```python
from build123d import *

# Parameters (mm, degrees)
BOSS_EXTRUDE1_DEPTH = 10
SKETCH2_R           = 10
BOSS_EXTRUDE2_DEPTH = 50
FILLET1_R           = 3
CHAMFER1_SIZE       = 2


with BuildPart() as part:
    # Sketch1 → Boss-Extrude1 (new body)
    with BuildSketch(Plane.XY):
        with BuildLine():
            Line((0, 20), (50, 20))
            ThreePointArc((50, 20), (70, 0), (50, -20))
            Line((50, -20), (0, -20))
            ThreePointArc((0, -20), (-20, 0), (0, 20))
        make_face()
        with BuildLine():
            Line((9.539392014, 3), (12, 3))
            Line((12, 3), (12, -3))
            Line((12, -3), (9.539392014, -3))
            ThreePointArc((9.539392014, -3), (-10, 0), (9.539392014, 3))
        make_face(mode=Mode.SUBTRACT)
    extrude(amount=BOSS_EXTRUDE1_DEPTH)

    # Sketch2 → Boss-Extrude2 (add)
    with BuildSketch(Plane.XY.offset(10)):
        with Locations((50, 0)):
            Circle(SKETCH2_R)
    extrude(amount=BOSS_EXTRUDE2_DEPTH)

    # Fillet1
    fillet1_edges = [part.edges().sort_by_distance(p)[0] for p in [
        (40, 0, 60),
    ]]
    fillet(fillet1_edges, radius=FILLET1_R)

    # Chamfer1
    chamfer1_edges = [part.edges().sort_by_distance(p)[0] for p in [
        (70, 0, 10),
        (25, 20, 10),
        (-20, 0, 10),
        (25, -20, 10),
    ]]
    chamfer(chamfer1_edges, length=CHAMFER1_SIZE)


solid = part.part
```
Design review of the part built by this model. Coordinates are the model's own, in mm. A direction names the side the tool comes from. Coordinates: 2 decimals unless noted, no trailing zeros. Order: outer loops, then holes, each group sorted by start corner. A loop starts at its lowest first (then second) coordinate and runs counter-clockwise, first axis right, second up. Notation, with made-up numbers: (87, 40.25) - (97, 40.25) arc R7 ccw to (97, 44.25) - close; hole circle Ø2 at (59, -22). An arc over 180 degrees is marked (long way). Answer in a Markdown table with one row per item.
(1) Wall thickness on line 1 along X through (y, z) = (0, 5); line 2 along Y through (x, z) = (0, 6); line 3 along Z through (x, y) = (27, 4.5): over which ranges is each line inside the solid? List them lowest first. Write a range as from..to.
Checked values:
| item | result |
|---|---|
| line 1 | -20..-10, 12..70 |
| line 2 | -20..-10, 10..20 |
| line 3 | 0..10 |
(2) Consider section A-A on y = 0. State the section outline as (x, z) points.
Checked values:
| item | result |
|---|---|
| outline | (-20, 0) - (-10, 0) - (-10, 10) - (-18, 10) - (-20, 8) - close; (12, 0) - (70, 0) - (70, 8) - (68, 10) - (60, 10) - (60, 57) arc R3 ccw to (57, 60) - (43, 60) arc R3 ccw to (40, 57) - (40, 10) - (12, 10) - close |
(3) Clearance check with flat-ended pins moving along their axes: pin 1 (1.5 mm diameter, centred on y = -6.5, z = 41, fed in from +X); pin 2 (11 mm diameter, centred on x = 31, y = -3.5, fed in from +Z); pin 3 (2 mm diameter, centred on y = -3, z = 27, fed in from +X). State where each tip first meets the part, or that it passes through.
Checked values:
| item | result |
|---|---|
| pin 1 | x = 58.18 |
| pin 2 | z = 10 |
| pin 3 | x = 59.8 |
(4) Consider section D-D on z = 42.5. State the section outline as (x, y) points.
Checked values:
| item | result |
|---|---|
| outline | circle Ø20 at (50, 0) |
(5) Consider section B-B on x = 8. State the section outline as (y, z) points, plus the area to 3 significant figures.
Checked values:
| item | result |
|---|---|
| outline | (-20, 0) - (-6, 0) - (-6, 10) - (-18, 10) - (-20, 8) - close; (6, 0) - (20, 0) - (20, 8) - (18, 10) - (6, 10) - close |
| area | 276 mm^2 |
(6) For faces 5 (the cylindrical face through (-20, 0, 4)), 6 (the flat face through (11, -3, 5)), 7 (the cylindrical face through (40, 0, 33)), list the 3-axis set-ups (+Z, -Z, +X, -X, +Y, -Y) from which the entire face can be reached by the end or side of a thin tool; tool diameter is ignored.
Checked values:
| item | result |
|---|---|
| face 5 | +Z, -Z, -X |
| face 6 | +Z, -Z |
| face 7 | +Z |
(7) Consider section C-C on x = 30. State the section outline as (y, z) points.
Checked values:
| item | result |
|---|---|
| outline | (-20, 0) - (20, 0) - (20, 8) - (18, 10) - (-18, 10) - (-20, 8) - close |
(8) The part is to be moulded in two halves that separate along Y. For faces 1 (the flat face through (25, -19, 9)), 2 (the flat face through (26, 0, 0)), 3 (the conical face through (68.121, 0.399, 9.875)), 4 (the flat face through (11, 3, 5)), say which applies: released by +Y, released by -Y, zero draft, split by the parting line, or undercut.
Checked values:
| item | result |
|---|---|
| face 1 | released by -Y |
| face 2 | zero draft |
| face 3 | split by the parting line |
| face 4 | undercut |
